Check sheet for the drawn part. Datum: minimum x, y, z corner. Units: mm. A direction names the side the tool comes from. Round coordinates to 2 decimals unless told otherwise and drop trailing zeros. Write each loop counter-clockwise with the first axis right and the second up, starting at its lowest first coordinate (ties: lowest second). Pieces come first, ordered by that corner, then holes. Notation, with made-up numbers: M -1,39 L 58,39 A8 ccw 58,44 Z; hole C -28,8.5 d9. An arc over 180 degrees is marked long. One line per item, written item: value. Start each with the question number.
Item 1: Thickness scan on probe 1 along X at (y, z) = (28.5, 8); probe 2 along Y at (x, z) = (2.5, 2.5); probe 3 along X at (y, z) = (5.5, 4.25). Record the ranges inside material, lowest first. Write a range as from..to.
Item 2: Section check A-A, the plane y = 32. Record the cut outline in (x, z).
Item 3: Gauge pin test, flat ends, axial feed: pin 1 (2 mm diameter, centred on y = 21, z = 18.5, fed in from -X); pin 2 (2 mm diameter, centred on x = 4, z = 20.5, fed in from -Y); pin 3 (1 mm diameter, centred on y = 11.5, z = 5, fed in from +X). Record the tip position at first contact, or that the pin passes through.
Item 4: Section check D-D, the plane y = 22.5. Record the cut outline in (x, z), then the cut area to 3 significant figures.
Item 5: Tool access check on the marked faces 1 and 2. Record the directions out of +Z, -Z, +X, -X, +Y, -Y that give a thin tool (end or side, any length) a straight path to the whole face; none if there is none.
Item 6: Draft check along X on the marked faces 3, 4, 5 and 6. Enter one of: +X half, -X half, draft (parallel to the pull), parting line (faces both ways), or undercut.
Item 7: Section check C-C, the plane x = 18.75. Record the cut outline in (y, z).
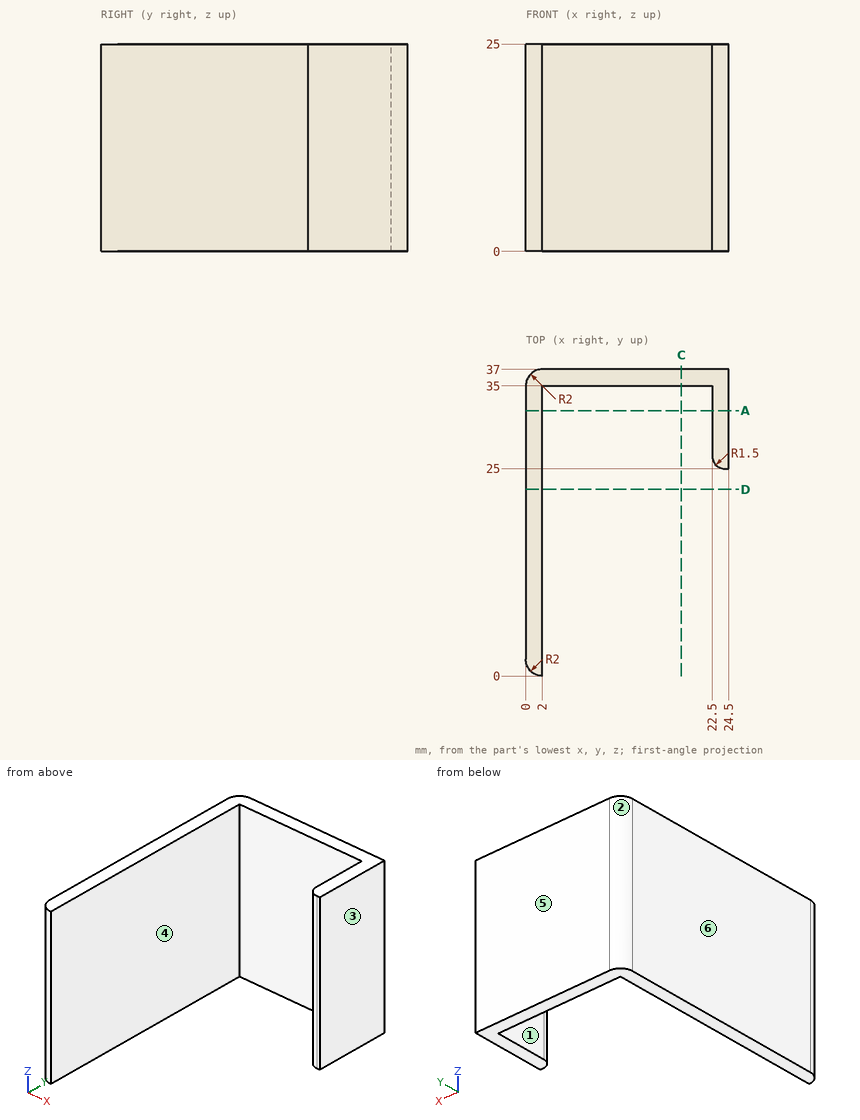
Response values:
1. probe 1: x = 0..2, 22.5..24.5
1. probe 2: y = 35..37
1. probe 3: x = 0..2
2. outline: M 0,0 L 2,0 L 2,25 L 0,25 Z; M 22.5,0 L 24.5,0 L 24.5,25 L 22.5,25 Z
3. pin 1: stops at x = 0
3. pin 2: stops at y = 35
3. pin 3: stops at x = 2
4. outline: M 0,0 L 2,0 L 2,25 L 0,25 Z
4. area: 50.0 mm2
5. face 1: +Z, -Z, -Y
5. face 2: +Z, -Z, -X, +Y
6. face 3: +X half
6. face 4: undercut
6. face 5: draft
6. face 6: -X half
7. outline: M 35,0 L 37,0 L 37,25 L 35,25 Z
